Autodesk Inventor part; units mm, degrees
ref_plane "YZ Plane" through (0, 0, 0) normal (1, 0, 0) x (0, 1, 0)
ref_plane "XZ Plane" through (0, 0, 0) normal (0, 1, 0) x (-1, 0, 0)
ref_plane "XY Plane" through (0, 0, 0) normal (0, 0, 1) x (1, 0, 0)
sketch "Sketch1" plane through (0, 0, 0) normal (0, 1, 0) x (-1, 0, 0)
  line L0 (150, 32.4) -> (-150, 32.4)
  line L1 (-150, 32.4) -> (-150, -32.4)
  line L2 (-150, -32.4) -> (150, -32.4)
  line L3 (150, -32.4) -> (150, 32.4)
  line L4 (150, 32.4) -> (-150, -32.4) construction
  line L5 (-150, 32.4) -> (150, -32.4) construction
  line L6 (160, 42.4) -> (-160, 42.4)
  line L7 (-160, 42.4) -> (-160, -42.4)
  line L8 (-160, -42.4) -> (160, -42.4)
  line L9 (160, -42.4) -> (160, 42.4)
  point P0 (0, 0)
  dimension "d0" = 64.8
  dimension "d1" = 300
  dimension "d2" = 10
  dimension "d15" = 84.8
extrude "Extrusion1" add sketch "Sketch1" along normal blind 10 contours L3 L2 L1 L0
extrude "Extrusion2" add sketch "Sketch1" along normal blind 50
sketch "Sketch2" plane through (160, 0, -42.4) normal (0, 0, -1) x (-1, 0, 0)
  point P0 (160, 0)
sketch "Sketch6" plane through (160, 0, -42.4) normal (0, 0, -1) x (-1, 0, 0)
  point P0 (160, 0)
sketch "Sketch7" plane through (160, 0, -42.4) normal (0, 0, -1) x (-1, 0, 0)
  point P0 (160, 0)
sketch "Sketch8" plane through (160, 0, -42.4) normal (0, 0, -1) x (-1, 0, 0)
  circle A0 centre (6.35, 4.7625) radius 3.175
  point P0 (160, 0)
  dimension "d12" = 6.35
extrude "Extrusion5" cut sketch "Sketch8" along normal mid plane 1000
properties part number "GiveBox"
Verification items for the finished model (mm, model axes). A direction names the side the tool comes from. Coordinates: 2 decimals unless noted, no trailing zeros. Write each loop counter-clockwise with the first axis right and the second up, starting at its lowest first coordinate (ties: lowest second). Pieces come first, ordered by that corner, then holes. Notation, with made-up numbers: M 53,51.5 L 85,51.5 A34 ccw 85,83.5 Z; hole C -12,-23 d9. An arc over 180 degrees is marked long. Answer as a JSON object with one key per item and string values. Group by question number.
(1) Cross-section at A-A, the plane x = 153.65. Record the cut outline in (y, z).
(2) Gauge pin test, flat ends, axial feed: pin 1 (12 mm diameter, centred on x = 32.5, z = 29.5, fed in from +Y); pin 2 (10 mm diameter, centred on x = -5, z = 3, fed in from +Y); pin 3 (5.5 mm diameter, centred on x = 153.65, y = 4.76, fed in from -Z). Record the tip position at first contact, or that the pin passes through.
(3) Cross-section at D-D, the plane x = -33. Record the cut outline in (y, z).
(4) Material ranges on line 1 (Z direction, x = 145.5, y = 35); line 2 (X direction, y = 25, z = -5); line 3 (Y direction, x = 153.65, z = -11.5), recorded low to high.
(5) Tool access check on faces 4 (the face through (2, 10, 0)), 5 (the face through (150.717, 3.546, -0.594)). Record the directions out of +Z, -Z, +X, -X, +Y, -Y that give a thin tool (end or side, any length) a straight path to the whole face; none if there is none.
(6) Release check for a two-part mould opening along Z. For faces 1 (the face through (2, 25, -42.4)), 2 (the face through (150, 30, 0)), 3 (the face through (-160, 25, -1)) record: +Z half, -Z half, draft (parallel to the pull), parting line (faces both ways), or undercut.
(7) Cross-section at B-B, the plane y = 19.5. Record the cut outline in (x, z).
Reply:
{
 "1": {"outline": "M 0,-42.4 L 1.59,-42.4 L 1.59,42.4 L 0,42.4 Z; M 7.94,-42.4 L 50,-42.4 L 50,42.4 L 7.94,42.4 Z"},
 "2": {"pin 1": "y = 50", "pin 2": "y = 10", "pin 3": "through"},
 "3": {"outline": "M 0,-42.4 L 50,-42.4 L 50,-32.4 L 10,-32.4 L 10,32.4 L 50,32.4 L 50,42.4 L 0,42.4 Z"},
 "4": {"line 1": "-42.4 to -32.4, 32.4 to 42.4", "line 2": "-160 to -150, 150 to 160", "line 3": "0 to 1.59, 7.94 to 50"},
 "5": {"face 4": "+Y", "face 5": "+Z, -Z"},
 "6": {"face 1": "-Z half", "face 2": "undercut", "face 3": "draft"},
 "7": {"outline": "M -160,-42.4 L 160,-42.4 L 160,42.4 L -160,42.4 Z; hole M -150,-32.4 L 150,-32.4 L 150,32.4 L -150,32.4 Z"}
}
